For this review, take the finished solid that the model builds, in its own axes (mm). A direction names the side the tool comes from. Give positions to 0.01 mm unless a question says otherwise; leave off trailing zeros. Order: outer loops, then holes, each group sorted by start corner. A loop starts at its lowest first (then second) coordinate and runs counter-clockwise, first axis right, second up.
Item 1: Consider section A-A (x = -65). Give the boundary of the cut face in (y, z), plus the area to 3 significant figures.
Item 2: Machinability: for faces 4 (the flat face through (65, -95, 30)), 5 (the flat face through (31.137, -249.65, 9.821)), 6 (the flat face through (-2, -186.411, 67)), 7 (the flat face through (-19.418, -249.65, -26.248)), 8 (the flat face through (0, -250, 32.648)), which of the approach directions +Z, -Z, +X, -X, +Y, -Y give a long, thin tool a straight path to every point of the face, cutting with its end or side? Answer none if there is none.
Item 3: For P1, Ø25, axis at y = -194, z = 72.5, coming from the +X side; P2, Ø10.5, axis at x = 59, y = -151.5, coming from the +Z side; P3, Ø2, axis at x = -23.5, y = -168, coming from the +Z side; P4, Ø1.5, axis at y = -128.5, z = 45.5, coming from the +X side, all flat-tipped, find the tip position at first contact; note any pin that passes through.
Item 4: Consider section B-B (y = -145). Give the boundary of the cut face in (x, z).
Item 5: For probe 1 along Y at (x, z) = (-65, 45.75); probe 2 along Y at (x, z) = (65, 36.25); probe 3 along Z at (x, y) = (17.5, -62), list the stretches that pass through material, from the lowest coordinate up.
Item 6: Consider section C-C (x = 105). Give the boundary of the cut face in (y, z), plus the area to 3 significant figures.
Item 7: Consider section D-D (y = -37). Give the boundary of the cut face in (x, z), plus the area to 3 significant figures.
Item 8: The part is to be moulded in two halves that separate along X. For faces 1 (the flat face through (-28, -220, -29)), 2 (the cylindrical face through (-55.592, -130.244, 40.14)), 3 (the flat face through (120, -202, 67)), say which applies: released by +X, released by -X, zero draft, split by the parting line, or undercut.
```python
from build123d import *

# Parameters (mm, degrees)
F0_W        = 250
F0_H        = 100
F1_DEPTH    = 220
F2_R        = 5
F4_DEPTH    = 60
F5_W        = 240
F5_H        = 28.5892599821
F6_DEPTH    = 40
F7_T1_DEPTH = 240
F7_T3_DEPTH = 265
F7_T5_DEPTH = 53.5892599821
F8_R        = 5
F9_R        = 17.5
F10_DEPTH   = 20


# Not quite as in the source:
# - a fillet or chamfer that OpenCascade refuses, or shapes differently, is made with other operations: its cross-section is extruded or revolved along the edge and cut away or added


with BuildPart() as f1:
    # F0 (on Front) → F1 (new body)
    with BuildSketch(Plane.XZ):
        Rectangle(F0_W, F0_H)
    extrude(amount=F1_DEPTH)

    # F2
    f2_edges = [f1.edges().sort_by_distance(p)[0] for p in [
        (125, -110, 50),
        (-125, -110, 50),
        (0, 0, 50),
        (0, -220, 50),
        (-125, -110, -50),
        (125, -110, -50),
        (0, 0, -50),
        (0, -220, -50),
        (125, -220, 0),
        (-125, -220, 0),
        (-125, 0, 0),
        (125, 0, 0),
    ]]
    fillet(f2_edges, radius=F2_R)

    # F3 (on face) → F4 (join)
    with BuildSketch(Plane.XZ.offset(220)):
        Polygon((23.7203992628, 32.6483286917), (-23.7203992628, 32.6483286917), (-38.380412234, -12.4705518844), (0, -40.3555536147), (38.380412234, -12.4705518844), align=None)
    extrude(amount=F4_DEPTH)

    # F5 (on face) → F6 (join)
    with BuildSketch(Plane.XY.offset(50)):
        with Locations((0, -200.7053700089)):
            Rectangle(F5_W, F5_H)
    extrude(amount=F6_DEPTH)

    # F7: fillet of radius 5 on 6 edges, made by hand

    # F7_s2 → F7_t1 (join)
    with BuildSketch(Plane.YZ.offset(-120)):
        with BuildLine():
            ThreePointArc((-217.5, 49.3301270189), (-215.6698729811, 51.1602540378), (-215, 53.6602540378))
            Line((-215, 53.6602540378), (-215, 50))
            ThreePointArc((-215, 50), (-216.2940952255, 49.8296291314), (-217.5, 49.3301270189))
        make_face()
    extrude(amount=F7_T1_DEPTH)

    # F7_s4 → F7_t3 (cut)
    with BuildSketch(Plane.YZ.offset(-132.5)):
        with BuildLine():
            ThreePointArc((-186.4107400179, 85), (-187.875206112, 88.5355339059), (-191.4107400179, 90))
            Line((-191.4107400179, 90), (-186.4107400179, 90))
            Line((-186.4107400179, 90), (-186.4107400179, 85))
        make_face()
        with BuildLine():
            ThreePointArc((-215, 85), (-213.5355339059, 88.5355339059), (-210, 90))
            Line((-210, 90), (-215, 90))
            Line((-215, 90), (-215, 85))
        make_face()
    extrude(amount=F7_T3_DEPTH, mode=Mode.SUBTRACT)

    # F7_s6 → F7_t5 (cut)
    with BuildSketch(Plane.XZ.offset(173.9107400179)):
        with BuildLine():
            ThreePointArc((-120, 85), (-118.5355339059, 88.5355339059), (-115, 90))
            Line((-115, 90), (-120, 90))
            Line((-120, 90), (-120, 85))
        make_face()
        with BuildLine():
            ThreePointArc((120, 85), (118.5355339059, 88.5355339059), (115, 90))
            Line((115, 90), (120, 90))
            Line((120, 90), (120, 85))
        make_face()
    extrude(amount=F7_T5_DEPTH, mode=Mode.SUBTRACT)

    # F8
    f8_edges = [f1.edges().sort_by_distance(p)[0] for p in [
        (0, -220, 32.648329),
        (31.050406, -220, 10.088888),
        (19.190206, -220, -26.413053),
        (-19.190206, -220, -26.413053),
        (-31.050406, -220, 10.088888),
        (31.050406, -280, 10.088888),
        (0, -280, 32.648329),
        (-31.050406, -280, 10.088888),
        (-19.190206, -280, -26.413053),
        (19.190206, -280, -26.413053),
        (-23.720399, -250, 32.648329),
        (23.720399, -250, 32.648329),
        (38.380412, -250, -12.470552),
        (0, -250, -40.355554),
        (-38.380412, -250, -12.470552),
    ]]
    fillet(f8_edges, radius=F8_R)

    # F9 (on face) → F10 (cut)
    with BuildSketch(Plane.XY.offset(50)):
        with Locations((-65, -45)):
            Circle(F9_R)
        with Locations((-65, -95)):
            Circle(F9_R)
        with Locations((-65, -145)):
            Circle(F9_R)
        with Locations((65, -145)):
            Circle(F9_R)
        with Locations((65, -95)):
            Circle(F9_R)
        with Locations((65, -45)):
            Circle(F9_R)
    extrude(amount=-F10_DEPTH, mode=Mode.SUBTRACT)


solid = f1.part
```
Resolved:
1. outline: (-220, -45) arc R5 ccw to (-215, -50) - (-5, -50) arc R5 ccw to (0, -45) - (0, 45) arc R5 ccw to (-5, 50) - (-27.5, 50) - (-27.5, 30) - (-62.5, 30) - (-62.5, 50) - (-77.5, 50) - (-77.5, 30) - (-112.5, 30) - (-112.5, 50) - (-127.5, 50) - (-127.5, 30) - (-162.5, 30) - (-162.5, 50) - (-186.41, 50) - (-186.41, 85) arc R5 ccw to (-191.41, 90) - (-210, 90) arc R5 ccw to (-215, 85) - (-215, 53.66) arc R5 cw to (-217.5, 49.33) arc R5 ccw to (-220, 45) - close
1. area: 21,000 mm2
2. face 4: +Z
2. face 5: +Z, +X, -Y
2. face 6: +Z, +X, -X, +Y
2. face 7: -Z, -X, -Y
2. face 8: +Z, +X, -X, -Y
3. P1: stops at x = 120
3. P2: stops at z = 30
3. P3: stops at z = 50
3. P4: stops at x = 125
4. outline: (-125, -45) arc R5 ccw to (-120, -50) - (120, -50) arc R5 ccw to (125, -45) - (125, 45) arc R5 ccw to (120, 50) - (82.5, 50) - (82.5, 30) - (47.5, 30) - (47.5, 50) - (-47.5, 50) - (-47.5, 30) - (-82.5, 30) - (-82.5, 50) - (-120, 50) arc R5 ccw to (-125, 45) - close
5. probe 1: y = -219.94 to -162.5, -127.5 to -112.5, -77.5 to -62.5, -27.5 to -0.06
5. probe 2: y = -220 to -162.5, -127.5 to -112.5, -77.5 to -62.5, -27.5 to 0
5. probe 3: z = -50 to 50
6. outline: (-220, -45) arc R5 ccw to (-215, -50) - (-5, -50) arc R5 ccw to (0, -45) - (0, 45) arc R5 ccw to (-5, 50) - (-186.41, 50) - (-186.41, 85) arc R5 ccw to (-191.41, 90) - (-210, 90) arc R5 ccw to (-215, 85) - (-215, 53.66) arc R5 cw to (-217.5, 49.33) arc R5 ccw to (-220, 45) - close
6. area: 23,100 mm2
7. outline: (-125, -45) arc R5 ccw to (-120, -50) - (120, -50) arc R5 ccw to (125, -45) - (125, 45) arc R5 ccw to (120, 50) - (80.56, 50) - (80.56, 30) - (49.44, 30) - (49.44, 50) - (-49.44, 50) - (-49.44, 30) - (-80.56, 30) - (-80.56, 50) - (-120, 50) arc R5 ccw to (-125, 45) - close
7. area: 23,700 mm2
8. face 1: zero draft
8. face 2: undercut
8. face 3: released by +X
